Read the model definition and answer for the solid it produces. Units are mm, in the model's axes. A direction names the side the tool comes from. Give positions to 0.01 mm unless a question says otherwise; leave off trailing zeros. Loops run counter-clockwise (first coordinate to the right, second up) from the corner with the lowest first, then second, coordinate; pieces in that order, holes last. Notation, with made-up numbers: (37, 27.5) - (73, 27.5) arc R19 ccw to (73, 48.5) - close; hole circle Ø4 at (-36, -39). An arc over 180 degrees is marked (long way). Write item = value, one per line.
Autodesk Inventor part; units mm, degrees
ref_plane "YZ Plane" through (0, 0, 0) normal (1, 0, 0) x (0, 1, 0)
ref_plane "XZ Plane" through (0, 0, 0) normal (0, 1, 0) x (-1, 0, 0)
ref_plane "XY Plane" through (0, 0, 0) normal (0, 0, 1) x (1, 0, 0)
sketch "Sketch1" plane through (0, 0, 0) normal (1, 0, 0) x (0, 1, 0)
  arc A0 (3.7123, 3.7123) -> (3.7123, -3.7123) centre (0, 0) ccw
  line L0 (-5.9108, 3.75) -> (-7.9108, 3.75)
  line L1 (-7.9108, -3.75) -> (-5.9108, -3.75)
  line L2 (3.7123, -3.7123) -> (4.9497, -4.9497)
  line L3 (3.7123, 3.7123) -> (4.9497, 4.9497)
  arc A1 (-5.9108, -3.75) -> (4.9497, -4.9497) centre (0, 0) ccw
  arc A2 (4.9497, 4.9497) -> (-5.9108, 3.75) centre (0, 0) ccw
  line L4 (4.9497, 4.9497) -> (0, 0) construction
  line L5 (0, 0) -> (4.9497, -4.9497) construction
  line L6 (-7.9108, 5) -> (-10.9108, 5)
  line L7 (-10.9108, -5) -> (-7.9108, -5)
  line L8 (-7.9108, -5) -> (-7.9108, -3.75)
  line L9 (-7.9108, 3.75) -> (-7.9108, 5)
  arc A3 (-10.9108, -5) -> (-10.9108, 5) centre (-35.8138, 0) ccw
  line L10 (-7.9108, 3.75) -> (-7.9108, -3.75) construction
  point P0 (-5.25, 0)
  point P1 (-13.9108, 0)
  point P2 (-7.9108, 4.375)
  point P3 (-7.9108, -4.375)
  point P4 (-7.9108, 0)
  dimension "d0" = 90
  dimension "d5" = 2
  dimension "d9" = 14
  dimension "d10" = 10.5
  dimension "d11" = 7.5
  dimension "d12" = 3
  dimension "d14" = 50.8
  dimension "d15" = 10
extrude "Extrusion1" add sketch "Sketch1" along normal blind 10
fillet "Fillet1" radius 0.5 6 edges at (5, -7.9108, -5) (5, 4.9497, -4.9497) (5, 4.9497, 4.9497) (5, 3.7123, 3.7123) (5, 3.7123, -3.7123) (5, -7.9108, 5)
chamfer "Chamfer1" distance 0.75 angle 45 2 edges at (5, -5.9108, 3.75) (5, -5.9108, -3.75)
properties part number "snap_grip"
1) The mould has two halves that part along Y. Classify faces 1 (the face through (4.93, -6.08, -4.05)), 2 (the face through (4.93, -10.414, 0.07)), 3 (the face through (5, -10, 5)): pulls with the +Y half, pulls with the -Y half, needs draft (parallel to the pull), parting line crosses it, or undercut.
Output:
face_1 = undercut
face_2 = pulls with the -Y half
face_3 = needs draft
2) Each of these flat-tipped pins is pushed along its axis until it touches: P1, Ø3, axis at x = 2, y = -4.5, coming from the -Z side; P2, Ø1.4, axis at x = 6, y = -7, coming from the +Z side; P3, Ø0.8, axis at x = 5.5, z = 4, coming from the +Y side. Where does it stop, or does it pass through?
Output:
P1 = -6.32
P2 = 3.94
P3 = 4.4
3) A cutting plane is placed at B-B on x = 1. Determine the outline of the cut face in (y, z).
Output:
outline = (-10.91, -5) - (-8.41, -5) arc R0.5 ccw to (-7.91, -4.5) - (-7.91, -3.75) - (-6.66, -3.75) - (-5.48, -4.36) arc R7 ccw to (4.55, -5.32) arc R0.5 ccw to (4.58, -4.58) - (4.05, -4.05) arc R0.5 ccw to (3.38, -4.02) arc R5.25 cw (long way) to (3.38, 4.02) arc R0.5 ccw to (4.05, 4.05) - (4.58, 4.58) arc R0.5 ccw to (4.55, 5.32) arc R7 ccw to (-5.48, 4.36) - (-6.66, 3.75) - (-7.91, 3.75) - (-7.91, 4.5) arc R0.5 ccw to (-8.41, 5) - (-10.91, 5) arc R25.4 cw to start
4) A cutting plane is placed at A-A on y = 0. Determine the outline of the cut face in (x, z).
Output:
outline = (0, -7) - (10, -7) - (10, -5.25) - (0, -5.25) - close; (0, 5.25) - (10, 5.25) - (10, 7) - (0, 7) - close
5) A cutting plane is placed at D-D on y = -7.25. Determine the outline of the cut face in (x, z).
Output:
outline = (0, -3.75) - (10, -3.75) - (10, 3.75) - (0, 3.75) - close
6) Find the intervals of material crossed by probe 1 along Z at (x, y) = (6, 0); probe 2 along Y at (x, z) = (5, -4); probe 3 along Z at (x, y) = (8, 2), in increasing order.
Output:
probe_1 = -7 to -5.25, 5.25 to 7
probe_2 = -10.73 to -7.91, -6.18 to -3.4, 3.4 to 3.99
probe_3 = -6.71 to -4.85, 4.85 to 6.71
7) A cutting plane is placed at C-C on z = 0. Determine the outline of the cut face in (x, y), then the cut area to 3 significant figures.
Output:
outline = (0, -10.41) - (10, -10.41) - (10, -5.25) - (0, -5.25) - close
area = 51.6 mm²
8) A tool of negligible diameter and unlimited length cuts with its end or side. For faces 4 (the face through (4.93, -5.247, -0.167)), 5 (the face through (5, -7, -3.75)), 6 (the face through (4.93, -6.08, 4.05)), 7 (the face through (5, -10, -5)), from which of +Z, -Z, +X, -X, +Y, -Y can it reach the whole face along a straight path? Write none if from no direction.
Output:
face_4 = +X, -X
face_5 = -Z, +X, -X
face_6 = +Z, +X, -X
face_7 = -Z, +X, -X, -Y
